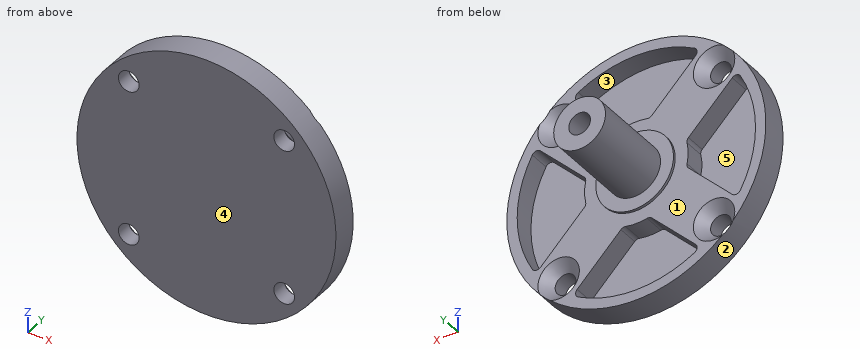
```python
from build123d import *

# Parameters (mm, degrees)
SKETCH_1_R             = 25
EXTRUDE_1_DEPTH        = 5
SKETCH_3_R             = 7.5
EXTRUDE_2_DEPTH        = 0.5
SKETCH_4_R             = 5
EXTRUDE_3_DEPTH        = 16
SKETCH_8_R             = 2
CUT_EXTRUDE_2_DEPTH    = 42.379342672
CHAMFER_1_SIZE         = 2
CUT_EXTRUDE_5_DEPTH    = 4
FILLET_1_R             = 1
HOLE_WIZARD_M5_1_D     = 4.2
HOLE_WIZARD_M5_1_DEPTH = 12.4
HOLE_WIZARD_M5_1_TIP   = 1.2618073


with BuildPart() as part:
    # 草图1 → 凸台-拉伸1 (new body)
    with BuildSketch(Plane(origin=(0, 0, 0), x_dir=(1, 0, 0), z_dir=(0, 1, 0))):
        with Locations(Location((0, 0, 0), (0, 0, 270))):
            Circle(SKETCH_1_R)
    extrude(amount=EXTRUDE_1_DEPTH)

    # 草图3 → 凸台-拉伸2 (add)
    with BuildSketch(Plane(origin=(0, 5, 0), x_dir=(1, 0, 0), z_dir=(0, 1, 0))):
        with Locations(Location((0, 0, 0), (0, 0, 270))):
            Circle(SKETCH_3_R)
    extrude(amount=EXTRUDE_2_DEPTH)

    # 草图4 → 凸台-拉伸3 (add)
    with BuildSketch(Plane(origin=(0, 5.5, 0), x_dir=(1, 0, 0), z_dir=(0, 1, 0))):
        with Locations(Location((0, 0, 0), (0, 0, 270))):
            Circle(SKETCH_4_R)
    extrude(amount=EXTRUDE_3_DEPTH)

    # 草图8 → 切除-拉伸2 (cut, through all)
    with BuildSketch(Plane(origin=(0, 0, 0), x_dir=(-1, 0, 0), z_dir=(0, -1, 0))):
        with Locations(Location((-15, -15, 0), (0, 0, 90))):
            Circle(SKETCH_8_R)
        with Locations(Location((15, -15, 0), (0, 0, 90))):
            Circle(SKETCH_8_R)
        with Locations(Location((15, 15, 0), (0, 0, 90))):
            Circle(SKETCH_8_R)
        with Locations(Location((-15, 15, 0), (0, 0, 90))):
            Circle(SKETCH_8_R)
    extrude(amount=-CUT_EXTRUDE_2_DEPTH, mode=Mode.SUBTRACT)

    # 倒角1
    # the kernel refuses this chamfer: 2 mm, written as the material it takes off along each edge
    with BuildSketch(Plane(origin=(15, 5, -15), x_dir=(0, 0, -1), z_dir=(-1, 0, 0))) as chamfer_1_piece_1:
        Polygon((2 + CHAMFER_1_SIZE, 0), (2, CHAMFER_1_SIZE), (2, 0), align=None)
    revolve(axis=Axis((15, 5, -15), (0, -1, 0)), mode=Mode.SUBTRACT)
    with BuildSketch(Plane(origin=(-15, 5, -15), x_dir=(0, 0, -1), z_dir=(-1, 0, 0))) as chamfer_1_piece_2:
        Polygon((2 + CHAMFER_1_SIZE, 0), (2, CHAMFER_1_SIZE), (2, 0), align=None)
    revolve(axis=Axis((-15, 5, -15), (0, -1, 0)), mode=Mode.SUBTRACT)
    with BuildSketch(Plane(origin=(-15, 5, 15), x_dir=(0, 0, -1), z_dir=(-1, 0, 0))) as chamfer_1_piece_3:
        Polygon((2 + CHAMFER_1_SIZE, 0), (2, CHAMFER_1_SIZE), (2, 0), align=None)
    revolve(axis=Axis((-15, 5, 15), (0, -1, 0)), mode=Mode.SUBTRACT)
    with BuildSketch(Plane(origin=(15, 5, 15), x_dir=(0, 0, -1), z_dir=(-1, 0, 0))) as chamfer_1_piece_4:
        Polygon((2 + CHAMFER_1_SIZE, 0), (2, CHAMFER_1_SIZE), (2, 0), align=None)
    revolve(axis=Axis((15, 5, 15), (0, -1, 0)), mode=Mode.SUBTRACT)

    # 草图13 → 切除-拉伸5 (cut)
    with BuildSketch(Plane(origin=(0, 5, 0), x_dir=(1, 0, 0), z_dir=(0, 1, 0))):
        with BuildLine():
            Line((-12.33897396, 19.410041772), (-2.588190451, 9.659258263))
            ThreePointArc((-2.588190451, 9.659258263), (0, 10), (2.588190451, 9.659258263))
            Line((2.588190451, 9.659258263), (12.33897396, 19.410041772))
            ThreePointArc((12.33897396, 19.410041772), (0, 23), (-12.33897396, 19.410041772))
        make_face()
        with BuildLine():
            Line((19.410041772, -12.33897396), (9.659258263, -2.588190451))
            ThreePointArc((9.659258263, -2.588190451), (10, 0), (9.659258263, 2.588190451))
            Line((9.659258263, 2.588190451), (19.410041772, 12.33897396))
            ThreePointArc((19.410041772, 12.33897396), (23, 0), (19.410041772, -12.33897396))
        make_face()
        with BuildLine():
            Line((-12.33897396, -19.410041772), (-2.588190451, -9.659258263))
            ThreePointArc((-2.588190451, -9.659258263), (0, -10), (2.588190451, -9.659258263))
            Line((2.588190451, -9.659258263), (12.33897396, -19.410041772))
            ThreePointArc((12.33897396, -19.410041772), (0, -23), (-12.33897396, -19.410041772))
        make_face()
        with BuildLine():
            Line((-19.410041772, 12.33897396), (-9.659258263, 2.588190451))
            ThreePointArc((-9.659258263, 2.588190451), (-10, 0), (-9.659258263, -2.588190451))
            Line((-9.659258263, -2.588190451), (-19.410041772, -12.33897396))
            ThreePointArc((-19.410041772, -12.33897396), (-23, 0), (-19.410041772, 12.33897396))
        make_face()
    extrude(amount=-CUT_EXTRUDE_5_DEPTH, mode=Mode.SUBTRACT)

    # 圆角1
    fillet_1_edges = [part.edges().sort_by_distance(p)[0] for p in [
        (12.33897396, 3, 19.410041772),
        (-12.33897396, 3, 19.410041772),
        (-2.588190451, 3, 9.659258263),
        (2.588190451, 3, 9.659258263),
        (19.410041772, 3, -12.33897396),
        (19.410041772, 3, 12.33897396),
        (9.659258263, 3, 2.588190451),
        (9.659258263, 3, -2.588190451),
        (-19.410041772, 3, 12.33897396),
        (-19.410041772, 3, -12.33897396),
        (-9.659258263, 3, -2.588190451),
        (-9.659258263, 3, 2.588190451),
        (-12.33897396, 3, -19.410041772),
        (12.33897396, 3, -19.410041772),
        (2.588190451, 3, -9.659258263),
        (-2.588190451, 3, -9.659258263),
    ]]
    fillet(fillet_1_edges, radius=FILLET_1_R)

    # M5 螺纹孔1
    with Locations(Plane(origin=(0, 21.5, 0), x_dir=(1, 0, 0), z_dir=(0, 1, 0))):
        with Locations((0, 0)):
            Hole(HOLE_WIZARD_M5_1_D / 2, depth=HOLE_WIZARD_M5_1_DEPTH)
            with Locations((0, 0, -(HOLE_WIZARD_M5_1_DEPTH + HOLE_WIZARD_M5_1_TIP / 2))):  # 118° drill point
                Cone(0, HOLE_WIZARD_M5_1_D / 2, HOLE_WIZARD_M5_1_TIP, mode=Mode.SUBTRACT)


solid = part.part
```
Geometry check sheet. Reference: the model listing, model coordinates, mm. Face numbers are marked on the shaded views. A direction names the side the tool comes from. Give positions to 0.01 mm unless a question says otherwise; leave off trailing zeros. Write each loop counter-clockwise with the first axis right and the second up, starting at its lowest first coordinate (ties: lowest second). Pieces come first, ordered by that corner, then holes. Notation, with made-up numbers: (39.25, 15.25) -> (78.25, 15.25) arc R36 cw to (78.25, 50.25) -> close; hole circle Ø6 at (34.25, 4.25). An arc over 180 degrees is marked (long way). Use one line per item in the form item = value.
Item 1: Sectioned sample at A-A on x = 15. Enter the section's corners in (y, z).
Results list:
outline = (0, -20) -> (5, -20) -> (5, -19) -> (3, -17) -> (0, -17) -> close; (0, -13) -> (3, -13) -> (5, -11) -> (5, -7.93) -> (1, -7.93) -> (1, 7.93) -> (5, 7.93) -> (5, 11) -> (3, 13) -> (0, 13) -> close; (0, 17) -> (3, 17) -> (5, 19) -> (5, 20) -> (0, 20) -> close
Item 2: Depth check by flat-ended pin: pin 1 Ø10 at (x, z) = (13, 18) entering from +Y; pin 2 Ø10 at (x, y) = (7, 13) entering from +Z; pin 3 Ø8 at (x, z) = (-6.5, -8) entering from +Y; pin 4 Ø5 at (x, z) = (-15, 15) entering from -Y. Enter the tip coordinate at first touch or a pass-through.
Results list:
pin_1 = 5
pin_2 = 4.58
pin_3 = 5.5
pin_4 = 0
Item 3: Sectioned sample at C-C on y = 2. Count the separate pieces of the cut face and the enclosed holes in it, plus the area to 3 significant figures.
Results list:
separate_pieces = 1
enclosed_holes = 8
area = 1,100 mm2
Item 4: Access from +Z, -Z, +X, -X, +Y, -Y to the whole of each face (thin tool, end or side, straight path). Record for the marked faces 4 and 5.
Results list:
face_4 = +Z, -Z, +X, -X, -Y
face_5 = +Y
Item 5: Scan lines: line 1 (X direction, y = 1.15, z = -15); line 2 (Y direction, x = 2.5, z = -7.5); line 3 (Y direction, x = -9, z = -16.5). Record each from-to range of solid material in increasing order.
Results list:
line_1 = -20 to -17, -13 to -7.93, 7.93 to 13, 17 to 20
line_2 = 0 to 5
line_3 = 0 to 1
Item 6: Sectioned sample at B-B on y = 12.75. Enter the section's corners in (x, z).
Results list:
outline = circle Ø10 at (0, 0); hole circle Ø4.2 at (0, 0)
Item 7: Sectioned sample at D-D on x = -21. Enter the section's corners in (y, z), plus the area to 3 significant figures.
Results list:
outline = (0, -13.56) -> (5, -13.56) -> (5, -9.38) -> (1, -9.38) -> (1, 9.38) -> (5, 9.38) -> (5, 13.56) -> (0, 13.56) -> close
area = 60.6 mm2
Item 8: Mould release check, pull along X, two halves, no side actions. Record for the marked faces 1, 2 and 3: released by +X, released by -X, zero draft, split by the parting line, or undercut.
Results list:
face_1 = zero draft
face_2 = split by the parting line
face_3 = undercut
